The figure shows three views and two pictorial views of one solid part (mm, origin at its lowest corner). Answer the questions. Coordinates: 2 decimals unless noted, no trailing zeros. Order: outer loops, then holes, each group sorted by start corner. A loop starts at its lowest first (then second) coordinate and runs counter-clockwise, first axis right, second up. Notation, with made-up numbers: (3.5, 70) -> (46.5, 70) arc R13 cw to (46.5, 88) -> close; hole circle Ø10 at (50, 3.25). An arc over 180 degrees is marked (long way). Write item = value, one per line. Start each with the question number.
Q1. The part is cut by section A-A, the plane z = 45. Determine the outline of the cut face in (x, y).
Q2. Straight lines are drawn through the part: L1, parallel to X at y = 20, z = 54; L2, parallel to Y at x = 45, z = 8. For each, find the intervals that lie inside material, in ascending order. Write a range as from..to.
Q3. For a pull along Y with two mould halves and no side action, classify the marked faces 1, 2 and 3 as +Y half, -Y half, draft (parallel to the pull), parting line (faces both ways), or undercut.
Q4. The part is cut by section B-B, the plane y = 32. Determine the outline of the cut face in (x, z).
Q5. Flat-ended cylindrical pins translate along their axes: pin 1 (6 mm diameter, centred on x = 18.5, z = 85.5, fed in from +Y); pin 2 (12 mm diameter, centred on y = 16.5, z = 39.5, fed in from -X). Find the tip coordinate at first contact, or state that the pin passes through.
Q6. The part is cut by section C-C, the plane x = 23. Determine the outline of the cut face in (y, z).
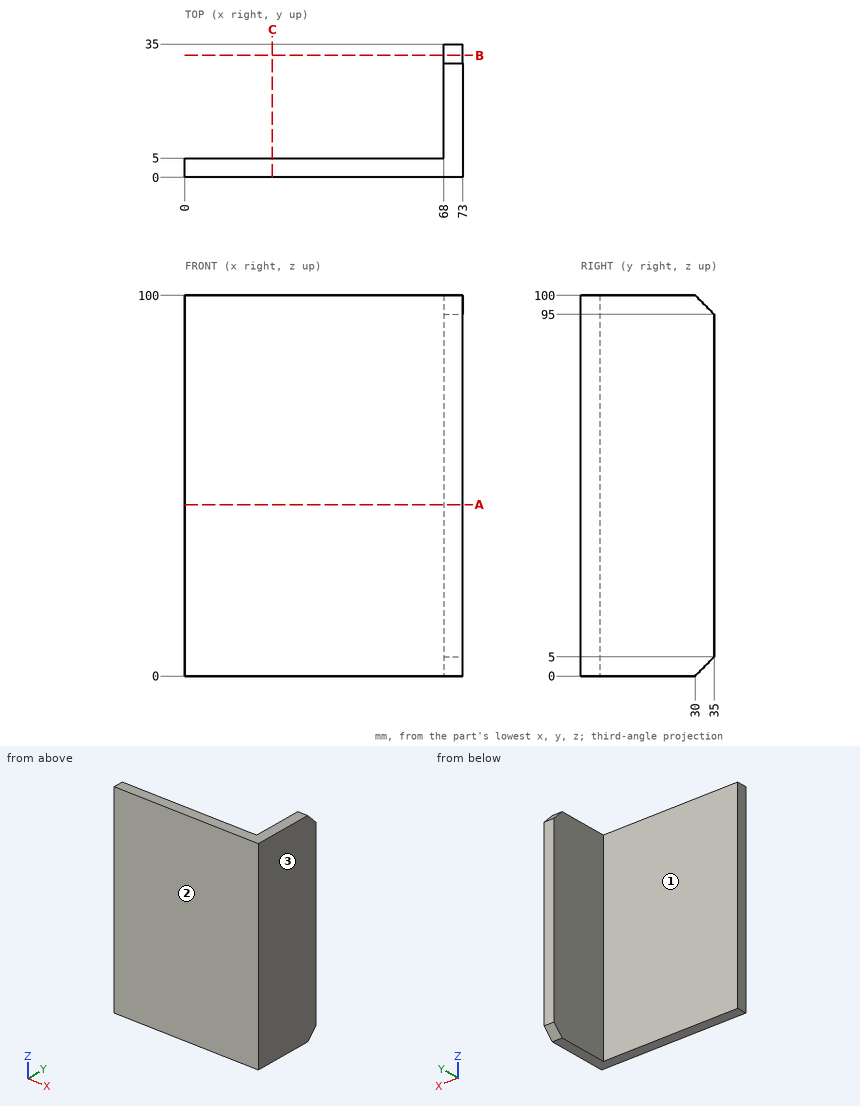
Model answer:
q1.outline = (0, 0) -> (73, 0) -> (73, 35) -> (68, 35) -> (68, 5) -> (0, 5) -> close
q2.L1 = 68..73
q2.L2 = 0..5
q3.face_1 = +Y half
q3.face_2 = -Y half
q3.face_3 = draft
q4.outline = (68, 2) -> (73, 2) -> (73, 98) -> (68, 98) -> close
q5.pin_1 = 5
q5.pin_2 = 68
q6.outline = (0, 0) -> (5, 0) -> (5, 100) -> (0, 100) -> close
